from build123d import *

# Parameters (mm, degrees)
SALIENTE_EXTRUIR1_DEPTH    = 40
CROQUIS2_R                 = 7.5
CORTAR_EXTRUIR1_DEPTH      = 40
CROQUIS3_R                 = 7.5
CORTAR_EXTRUIR2_DEPTH      = 40
CORTAR_EXTRUIR4_DEPTH      = 15
CORTAR_EXTRUIR4_DEPTH_BACK = 15


with BuildPart() as part:
    # Croquis1 → Saliente-Extruir1 (new body)
    with BuildSketch(Plane.XY):
        Polygon((0, 0), (140, 0), (140, 30), (115, 30), (100, 60), (40, 60), (25, 30), (0, 30), align=None)
    extrude(amount=SALIENTE_EXTRUIR1_DEPTH)

    # Croquis2 → Cortar-Extruir1 (cut)
    with BuildSketch(Plane(origin=(0, 30, 0), x_dir=(1, 0, 0), z_dir=(0, 1, 0))):
        with Locations((127.532427411, -19.421880323)):
            Circle(CROQUIS2_R)
    extrude(amount=-CORTAR_EXTRUIR1_DEPTH, mode=Mode.SUBTRACT)

    # Croquis3 → Cortar-Extruir2 (cut)
    with BuildSketch(Plane(origin=(0, 30, 0), x_dir=(1, 0, 0), z_dir=(0, 1, 0))):
        with Locations((12.5, -20)):
            Circle(CROQUIS3_R)
    extrude(amount=-CORTAR_EXTRUIR2_DEPTH, mode=Mode.SUBTRACT)

    # Croquis16 → Cortar-Extruir4 (cut, two sides)
    with BuildSketch(Plane(origin=(70, 0, 0), x_dir=(0, 0, -1), z_dir=(1, 0, 0))) as cortar_extruir4_sk:
        Polygon((0, 60), (-20, 60), (0, 25.358983849), align=None)
    extrude(amount=CORTAR_EXTRUIR4_DEPTH, mode=Mode.SUBTRACT)
    extrude(cortar_extruir4_sk.sketch, amount=-CORTAR_EXTRUIR4_DEPTH_BACK, mode=Mode.SUBTRACT)


solid = part.part
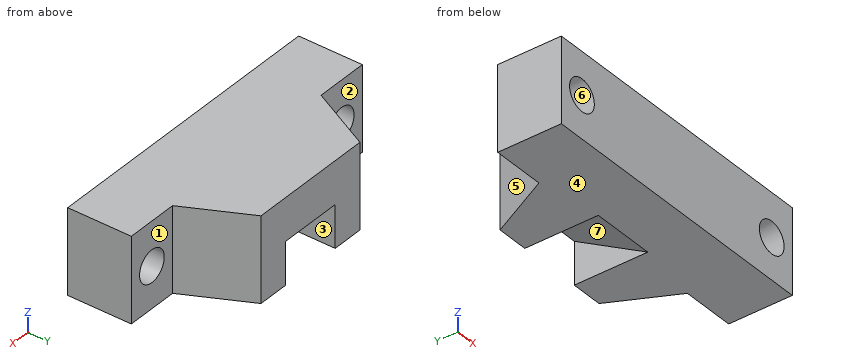
Input: part model. Units: mm. Frame: model coordinates. Face numbers are marked on the shaded views. A direction names the side the tool comes from. Coordinates: 2 decimals unless noted, no trailing zeros. Loops run counter-clockwise (first coordinate to the right, second up) from the corner with the lowest first, then second, coordinate; pieces in that order, holes last.
(1) Section A-A on x = 12.5. Return the cut outline in (y, z), then the cut area to 3 significant figures.
(2) Section B-B on y = 38. Return the cut outline in (x, z).
(3) Pull-direction query (Z, two-part tool) for the marked faces 5, 6 and 7; classes: released by +Z, released by -Z, zero draft, split by the parting line, or undercut.
(4) Section D-D on x = 74. Return the cut outline in (y, z), then the cut area to 3 significant figures.
(5) Set-up query: the marked faces 1, 2, 3 and 4. Return all of +Z, -Z, +X, -X, +Y, -Y with unobstructed straight access to the full face (end or side cutting, diameter ignored); none if empty.
(6) Section C-C on z = 9.5. Return the cut outline in (x, y).
(7) First-contact query: pin 1 Ø22 at (y, z) = (41.5, 11) entering from +X; pin 2 Ø12.5 at (x, z) = (124, 29) entering from +Y. Flat tips, straight axial feed; report the tip coordinate or a pass-through.
(8) Material intervals for probe 1 along X at (y, z) = (18.5, 20); probe 2 along Z at (x, y) = (12.5, 14.75); probe 3 along X at (y, z) = (19.5, 24.5), sorted ascending.
Data:
1. outline: (0, 0) - (30, 0) - (30, 12.5) - (0, 12.5) - close; (0, 27.5) - (30, 27.5) - (30, 40) - (0, 40) - close
1. area: 750 mm2
2. outline: (29, 0) - (55, 0) - (55, 7.3) - (85, 7.3) - (85, 0) - (111, 0) - (111, 40) - (29, 40) - close
3. face 5: zero draft
3. face 6: undercut
3. face 7: released by -Z
4. outline: (0, 0) - (25.36, 0) - (60, 20) - (60, 40) - (0, 40) - close
4. area: 2,050 mm2
5. face 1: +Z, -Z, +X, +Y
5. face 2: +Z, -Z, -X, +Y
5. face 3: -Z, +Y
5. face 4: -Z, +X, -X, +Y, -Y
6. outline: (0, 0) - (140, 0) - (140, 30) - (115, 30) - (100, 60) - (85, 60) - (85, 41.81) - (55, 41.81) - (55, 60) - (40, 60) - (25, 30) - (0, 30) - close
7. pin 1: stops at x = 114.75
7. pin 2: stops at y = 30
8. probe 1: x = 0 to 5, 20 to 120.05, 135.01 to 140
8. probe 2: z = 0 to 12.5, 27.5 to 40
8. probe 3: x = 0 to 6.5, 18.5 to 122.01, 133.05 to 140
